Model file for the job. Use its own axes, mm. A direction names the side the tool comes from. Coordinates: 2 decimals unless noted, no trailing zeros. Write each loop counter-clockwise with the first axis right and the second up, starting at its lowest first coordinate (ties: lowest second). Pieces come first, ordered by that corner, then holes. Notation, with made-up numbers: (56.5, 68) -> (81.5, 68) arc R20 ccw to (81.5, 107) -> close; hole circle Ø10 at (57, 13.25). An arc over 180 degrees is marked (long way). Write item = value, one per line. Start each with the question number.
from build123d import *

# Parameters (mm, degrees)
F1_DEPTH = 8
F2_R     = 2.5
F3_T     = -1.5


with BuildPart() as f1:
    # F0 (on Top) → F1 (new body)
    with BuildSketch(Plane.XY):
        with BuildLine():
            Line((40, 22.5), (-40, 22.5))
            ThreePointArc((-40, 22.5), (-43.535534, 21.035534), (-45, 17.5))
            Line((-45, 17.5), (-45, -17.5))
            ThreePointArc((-45, -17.5), (-43.535534, -21.035534), (-40, -22.5))
            Line((-40, -22.5), (40, -22.5))
            ThreePointArc((40, -22.5), (43.535534, -21.035534), (45, -17.5))
            Line((45, -17.5), (45, 17.5))
            ThreePointArc((45, 17.5), (43.535534, 21.035534), (40, 22.5))
        make_face()
        with BuildLine():
            ThreePointArc((-17.5, 8), (-16.914214, 9.414214), (-15.5, 10))
            Line((-15.5, 10), (15.5, 10))
            ThreePointArc((15.5, 10), (16.914214, 9.414214), (17.5, 8))
            Line((17.5, 8), (17.5, -8))
            ThreePointArc((17.5, -8), (16.914214, -9.414214), (15.5, -10))
            Line((15.5, -10), (-15.5, -10))
            ThreePointArc((-15.5, -10), (-16.914214, -9.414214), (-17.5, -8))
            Line((-17.5, -8), (-17.5, 8))
        make_face(mode=Mode.SUBTRACT)
    extrude(amount=F1_DEPTH)

    # F2
    f2_edges = [f1.edges().sort_by_distance(p)[0] for p in [
        (0, -22.5, 8),
    ]]
    fillet(f2_edges, radius=F2_R)

    # F3
    f3_openings = [f1.faces().sort_by_distance(p)[0] for p in [
        (0, 21.493769, 0),
    ]]
    offset(amount=F3_T, openings=f3_openings)


solid = f1.part
(1) Saw through at A-A (z = 3.75). State how many separate pieces and enclosed holes the cut face has, then the cut area to 3 significant figures.
(2) Drill centre lines: line 1 along X through (y, z) = (2, 3); line 2 along Y through (x, z) = (7, 1.5); line 3 along X through (y, z) = (9, 4.25). Where is each one in solid material? Low to high.
(3) 3-axis set-ups, long thin cutter, end or side, ignore diameter. For faces 4 (the face through (-42.5, -19.95, 2.71)), 5 (the face through (1, -22, 7)), 6 (the face through (0, 10, 4)): which of +Z, -Z, +X, -X, +Y, -Y reach the whole face in a straight line?
(4) Saw through at C-C (y = 14). Give the cut face in (x, z), then the cut area to 3 significant figures.
(5) Saw through at D-D (x = 26). Give the cut face in (y, z).
(6) Saw through at B-B (x = 6.5). Give the cut face in (y, z).
(7) Drop a flat-ended pin along its axis: pin 1 Ø12 at (x, y) = (32.5, -13.5) entering from -Z. Give the stop position or say it passes through.
(8) Mould opens along X. For faces 1 (the face through (-1, 14, 8)), 2 (the face through (-43.57, -21, 2.71)), 3 (the face through (16.93, -9.4, 3.94)) say: released by +X, released by -X, zero draft, split by the parting line, or undercut.
Returned:
q1.separate_pieces = 2
q1.enclosed_holes = 2
q1.area = 552 mm2
q2.line_1 = -45 to -43.5, -19 to -17.5, 17.5 to 19, 43.5 to 45
q2.line_2 = -22.5 to -21, -11.5 to -10, 10 to 11.5, 21 to 22.5
q2.line_3 = -45 to -43.5, -18.85 to -17.23, 17.23 to 18.85, 43.5 to 45
q3.face_4 = -Z
q3.face_5 = +Z, +X, -X, -Y
q3.face_6 = +Z, -Z
q4.outline = (-45, 0) -> (-43.5, 0) -> (-43.5, 5.5) arc R1 cw to (-42.5, 6.5) -> (42.5, 6.5) arc R1 cw to (43.5, 5.5) -> (43.5, 0) -> (45, 0) -> (45, 5.5) arc R2.5 ccw to (42.5, 8) -> (-42.5, 8) arc R2.5 ccw to (-45, 5.5) -> close
q4.area = 152 mm2
q5.outline = (-22.5, 0) -> (-21, 0) -> (-21, 5.5) arc R1 cw to (-20, 6.5) -> (20, 6.5) arc R1 cw to (21, 5.5) -> (21, 0) -> (22.5, 0) -> (22.5, 5.5) arc R2.5 ccw to (20, 8) -> (-20, 8) arc R2.5 ccw to (-22.5, 5.5) -> close
q6.outline = (-22.5, 0) -> (-21, 0) -> (-21, 5.5) arc R1 cw to (-20, 6.5) -> (-11.5, 6.5) -> (-11.5, 0) -> (-10, 0) -> (-10, 8) -> (-20, 8) arc R2.5 ccw to (-22.5, 5.5) -> close; (10, 0) -> (11.5, 0) -> (11.5, 6.5) -> (20, 6.5) arc R1 cw to (21, 5.5) -> (21, 0) -> (22.5, 0) -> (22.5, 5.5) arc R2.5 ccw to (20, 8) -> (10, 8) -> close
q7.pin_1 = 6.5
q8.face_1 = zero draft
q8.face_2 = released by -X
q8.face_3 = undercut
